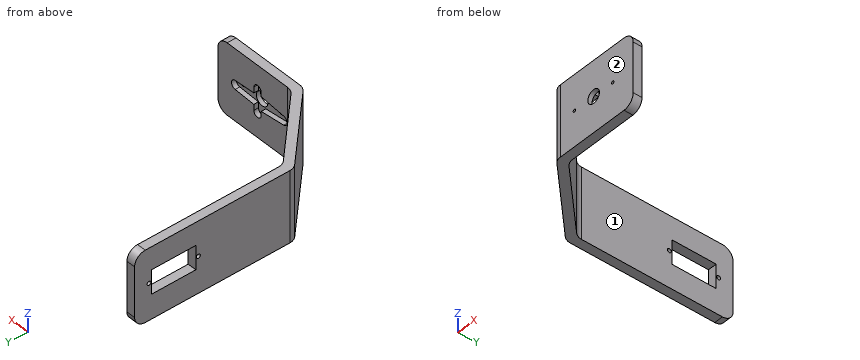
```python
from build123d import *

# Parameters (mm, degrees)
EXTRUDE_1_DEPTH     = 40
FILLET_7_R          = 6
CUT_EXTRUDE_4_DEPTH = 2.6
SKETCH_7_R          = 1.1
SKETCH_7_W          = 13.5
SKETCH_7_H          = 25
CUT_EXTRUDE_5_DEPTH = 10
FILLET_8_R          = 6
FILLET_9_R          = 6
FILLET_10_R         = 6
FILLET_11_R         = 6
FILLET_12_R         = 6
FILLET_13_R         = 6
FILLET_14_R         = 6
SKETCH_10_R         = 3.8
SKETCH_10_R_2       = 0.8
CUT_EXTRUDE_7_DEPTH = 10


with BuildPart() as part:
    # 草图1 → 凸台-拉伸1 (new body)
    with BuildSketch(Plane.XY):
        Polygon((15.872975722, -72.274332462), (-32.055956466, -72.274332462), (-67.411295525, -36.918993403), (-67.411295525, 51.009938785), (-72.411295525, 51.009938785), (-72.411295525, -38.990061215), (-34.127024278, -77.274332462), (15.872975722, -77.274332462), align=None)
    extrude(amount=EXTRUDE_1_DEPTH)

    # 圆角7
    fillet_7_edges = [part.edges().sort_by_distance(p)[0] for p in [
        (-34.127024278, -77.274332462, 20),
    ]]
    fillet(fillet_7_edges, radius=FILLET_7_R)

    # 草图6 → 切除-拉伸4 (cut)
    with BuildSketch(Plane(origin=(0, -72.274332462, 0), x_dir=(1, 0, 0), z_dir=(0, 1, 0))):
        with BuildLine():
            Line((4.635801051, -17.503483429), (-7.546126997, -16.859731248))
            Line((-7.546126997, -16.859731248), (-7.546126997, -13.55))
            ThreePointArc((-7.546126997, -13.55), (-9.946126997, -11.15), (-12.346126997, -13.55))
            Line((-12.346126997, -13.55), (-12.346126997, -15.950319654))
            Line((-12.346126997, -15.950319654), (-27.060314717, -17.51399822))
            ThreePointArc((-27.060314717, -17.51399822), (-29.296126997, -20), (-27.060314717, -22.48600178))
            Line((-27.060314717, -22.48600178), (-12.346126997, -24.049680346))
            Line((-12.346126997, -24.049680346), (-12.346126997, -26.45))
            ThreePointArc((-12.346126997, -26.45), (-9.946126997, -28.85), (-7.546126997, -26.45))
            Line((-7.546126997, -26.45), (-7.546126997, -23.140268752))
            Line((-7.546126997, -23.140268752), (4.635801051, -22.496516571))
            ThreePointArc((4.635801051, -22.496516571), (7.003873003, -20), (4.635801051, -17.503483429))
        make_face()
    extrude(amount=-CUT_EXTRUDE_4_DEPTH, mode=Mode.SUBTRACT)

    # 草图7 → 切除-拉伸5 (cut)
    with BuildSketch(Plane(origin=(-67.411295525, -6.360766816, 0), x_dir=(0, 0, -1), z_dir=(-1, 0, 0))):
        with Locations((-20.5, -49.239005853)):
            Circle(SKETCH_7_R)
        with Locations((-20.5, -21.439005853)):
            Circle(SKETCH_7_R)
        with Locations((-20.5, -35.339005853)):
            Rectangle(SKETCH_7_W, SKETCH_7_H)
    extrude(amount=CUT_EXTRUDE_5_DEPTH, mode=Mode.SUBTRACT)

    # 圆角8
    fillet_8_edges = [part.edges().sort_by_distance(p)[0] for p in [
        (-32.055956466, -72.274332462, 20),
    ]]
    fillet(fillet_8_edges, radius=FILLET_8_R)

    # 圆角9
    fillet_9_edges = [part.edges().sort_by_distance(p)[0] for p in [
        (-72.411295525, -38.990061215, 20),
    ]]
    fillet(fillet_9_edges, radius=FILLET_9_R)

    # 圆角10
    fillet_10_edges = [part.edges().sort_by_distance(p)[0] for p in [
        (-67.411295525, -36.918993403, 20),
    ]]
    fillet(fillet_10_edges, radius=FILLET_10_R)

    # 圆角11
    fillet_11_edges = [part.edges().sort_by_distance(p)[0] for p in [
        (-69.911295525, 51.009938785, 0),
    ]]
    fillet(fillet_11_edges, radius=FILLET_11_R)

    # 圆角12
    fillet_12_edges = [part.edges().sort_by_distance(p)[0] for p in [
        (-69.911295525, 51.009938785, 40),
    ]]
    fillet(fillet_12_edges, radius=FILLET_12_R)

    # 圆角13
    fillet_13_edges = [part.edges().sort_by_distance(p)[0] for p in [
        (15.872975722, -74.774332462, 0),
    ]]
    fillet(fillet_13_edges, radius=FILLET_13_R)

    # 圆角14
    fillet_14_edges = [part.edges().sort_by_distance(p)[0] for p in [
        (15.872975722, -74.774332462, 40),
    ]]
    fillet(fillet_14_edges, radius=FILLET_14_R)

    # 草图10 → 切除-拉伸7 (cut)
    with BuildSketch(Plane(origin=(0, -74.874332462, 0), x_dir=(1, 0, 0), z_dir=(0, 1, 0))):
        with Locations(Location((-9.946126997, -20, 0), (0, 0, 180))):
            Circle(SKETCH_10_R)
        with Locations(Location((2.553873003, -20, 0), (0, 0, 180))):
            Circle(SKETCH_10_R_2)
        with Locations(Location((-22.446126997, -20, 0), (0, 0, 270))):
            Circle(SKETCH_10_R_2)
    extrude(amount=-CUT_EXTRUDE_7_DEPTH, mode=Mode.SUBTRACT)


solid = part.part
```
Source: CAD feature listing. Evaluate the final solid. Frame: model axes, mm. Face numbers are marked on the shaded views. A direction names the side the tool comes from. Coordinates: 2 decimals unless noted, no trailing zeros. Write each loop counter-clockwise with the first axis right and the second up, starting at its lowest first coordinate (ties: lowest second). Pieces come first, ordered by that corner, then holes. Notation, with made-up numbers: M 34.25,85.25 L 55.25,85.25 A23 ccw 55.25,94.25 Z; hole C 36.5,-33.5 d7. An arc over 180 degrees is marked long. Answer as a JSON object with one key per item and string values.
1. Cut plane C-C on x = -53. Output: boundary loops of the cut face in (y, z).
Evaluation:
{"outline": "M -58.4,0 L -51.33,0 L -51.33,40 L -58.4,40 Z"}
2. Access query for the marked faces 1 and 2. Directions: +Z, -Z, +X, -X, +Y, -Y. A direction counts if a zero-diameter tool reaches every point of the face in a straight line with its end or side. Return the directions, or none.
Evaluation:
{"face 1": "+Z, -Z, +X, +Y", "face 2": "+Z, -Z, +X, -X, -Y"}
3. Contact query for flat-ended pins moving along their axis: P1, Ø1.3, axis at y = -73.5, z = 15, coming from the -X side; P2, Ø1, axis at x = -4, z = 24, coming from the +Y side; P3, Ø4, axis at y = 26.5, z = 10, coming from the +X side; P4, Ø7, axis at x = -9.95, z = 20, coming from the -Y side. Output: stop coordinate, or through.
Evaluation:
{"P1": "x = -38.55", "P2": "y = -72.27", "P3": "x = -67.41", "P4": "through"}
4. Cut plane A-A on y = -6.5. Output: boundary loops of the cut face in (x, z), plus the area to 3 significant figures.
Evaluation:
{"outline": "M -72.41,0 L -67.41,0 L -67.41,40 L -72.41,40 Z", "area": "200 mm^2"}
5. Ray query, L1, parallel to Y at x = -70.65, z = 20.5; L2, parallel to Y at x = -71, z = 20; L3, parallel to X at y = -22, z = 22. Return the intervals inside material, ascending.
Evaluation:
{"L1": "-40.75 to 13.98, 16.18 to 16.48, 41.48 to 41.78, 43.98 to 51.01", "L2": "-40.37 to 14.1, 16.06 to 16.48, 41.48 to 41.9, 43.86 to 51.01", "L3": "-72.41 to -67.41"}
6. Cut plane B-B on z = 4. Output: boundary loops of the cut face in (x, y), plus the area to 3 significant figures.
Evaluation:
{"outline": "M -72.41,-36.5 A6 ccw -70.65,-40.75 L -35.88,-75.52 A6 ccw -31.64,-77.27 L 15.53,-77.27 L 15.53,-72.27 L -29.57,-72.27 A6 cw -33.81,-70.52 L -65.65,-38.68 A6 cw -67.41,-34.43 L -67.41,50.67 L -72.41,50.67 Z", "area": "947 mm^2"}
